Geometry: final body of the model. Coordinates: model frame, mm. A direction names the side the tool comes from. Coordinates: 2 decimals unless noted, no trailing zeros. Order: outer loops, then holes, each group sorted by start corner. A loop starts at its lowest first (then second) coordinate and runs counter-clockwise, first axis right, second up. Notation, with made-up numbers: (35.5, 24) - (40.5, 24) arc R20 ccw to (40.5, 60) - close; hole circle Ø6 at (-36.75, -9.5). An arc over 180 degrees is marked (long way). Use a Markdown table: item, result. Add a question column.
```python
from build123d import *

# Parameters (mm, degrees)
BOSS_EXTRUDE1_DEPTH = 3.175
VARFILLET1_START    = -1
VARFILLET1_DEPTH    = 5
VARFILLET2_DEPTH    = 3.175
SKETCH5_R           = 25.4
CUT_EXTRUDE1_DEPTH  = 3.175
SKETCH5_11_R        = 26.9875
SKETCH5_11_R_2      = 25.4
CUT_EXTRUDE2_DEPTH  = 0.9906
SKETCH24_R          = 11.1125
SKETCH24_R_2        = 7.9375
CUT_EXTRUDE5_DEPTH  = 0.9906
SKETCH24_2_R        = 7.9375
CUT_EXTRUDE6_DEPTH  = 3.175
SKETCH32_R          = 3.175
SKETCH32_R_2        = 3.2639
CUT_EXTRUDE10_DEPTH = 3.175
CIRPATTERN1_COUNT   = 3


with BuildPart() as part:
    # Basic Outline → Boss-Extrude1 (new body)
    with BuildSketch(Plane.XY):
        with BuildLine():
            Line((-38.1, 98.7206881), (-38.1, 21.997045256))
            Line((-38.1, 21.997045256), (-104.544623774, -16.364776166))
            ThreePointArc((-104.544623774, -16.364776166), (-76.653488005, -44.255911934), (-66.444623774, -82.355911934))
            Line((-66.444623774, -82.355911934), (0, -43.994090512))
            Line((0, -43.994090512), (66.444623774, -82.355911934))
            ThreePointArc((66.444623774, -82.355911934), (76.653488005, -44.255911934), (104.544623774, -16.364776166))
            Line((104.544623774, -16.364776166), (38.1, 21.997045256))
            Line((38.1, 21.997045256), (38.1, 98.7206881))
            ThreePointArc((38.1, 98.7206881), (0, 88.511823868), (-38.1, 98.7206881))
        make_face()
    extrude(amount=BOSS_EXTRUDE1_DEPTH)

    # VarFillet1: read off the stored shape, not the designer's step
    # VarFillet1 outline → VarFillet1 (cut)
    with BuildSketch(Plane.XY.offset(VARFILLET1_START)):
        with BuildLine():
            Line((-38.1, 98.7206881), (-38.1, 93.43325065))
            add(Edge.make_bspline(
                [(-38.1, 93.43325065), (-38.1, 98.524577309), (-33.528, 96.284393579)],
                knots=[0, 0, 0, 1, 1, 1], degree=2, weights=[1, 0.529150262, 1]))
            ThreePointArc((-33.528, 96.284393579), (-35.83471053, 97.463675037), (-38.1, 98.7206881))
        make_face()
        with BuildLine():
            ThreePointArc((38.1, 98.7206881), (35.83471053, 97.463675037), (33.528, 96.284393579))
            add(Edge.make_bspline(
                [(33.528, 96.284393579), (38.1, 98.524577309), (38.1, 93.43325065)],
                knots=[0, 0, 0, 1, 1, 1], degree=2, weights=[1, 0.529150262, 1]))
            Line((38.1, 93.43325065), (38.1, 98.7206881))
        make_face()
        with BuildLine():
            add(Edge.make_bspline(
                [(-100.148730828, -19.106097052), (-104.374786847, -16.26672077), (-99.965568621, -13.721057441)],
                knots=[0, 0, 0, 1, 1, 1], degree=2, weights=[1, 0.529150262, 1]))
            Line((-99.965568621, -13.721057441), (-104.544623774, -16.364776166))
            ThreePointArc((-104.544623774, -16.364776166), (-102.323373793, -17.698067863), (-100.148730828, -19.106097052))
        make_face()
        with BuildLine():
            add(Edge.make_bspline(
                [(-61.865568621, -79.712193209), (-66.274786847, -82.257856539), (-66.620730828, -77.178296528)],
                knots=[0, 0, 0, 1, 1, 1], degree=2, weights=[1, 0.529150262, 1]))
            ThreePointArc((-66.620730828, -77.178296528), (-66.488663264, -79.765607174), (-66.444623774, -82.355911934))
            Line((-66.444623774, -82.355911934), (-61.865568621, -79.712193209))
        make_face()
        with BuildLine():
            Line((104.544623774, -16.364776166), (99.965568621, -13.721057441))
            add(Edge.make_bspline(
                [(99.965568621, -13.721057441), (104.374786847, -16.26672077), (100.148730828, -19.106097052)],
                knots=[0, 0, 0, 1, 1, 1], degree=2, weights=[1, 0.529150262, 1]))
            ThreePointArc((100.148730828, -19.106097052), (102.323373793, -17.698067863), (104.544623774, -16.364776166))
        make_face()
        with BuildLine():
            ThreePointArc((66.444623774, -82.355911934), (66.488663264, -79.765607174), (66.620730828, -77.178296528))
            add(Edge.make_bspline(
                [(66.620730828, -77.178296528), (66.274786847, -82.257856539), (61.865568621, -79.712193209)],
                knots=[0, 0, 0, 1, 1, 1], degree=2, weights=[1, 0.529150262, 1]))
            Line((61.865568621, -79.712193209), (66.444623774, -82.355911934))
        make_face()
    extrude(amount=VARFILLET1_DEPTH, mode=Mode.SUBTRACT)

    # VarFillet2: read off the stored shape, not the designer's step
    # VarFillet2 outline → VarFillet2 (add)
    with BuildSketch(Plane.XY):
        with BuildLine():
            add(Edge.make_bspline(
                [(6.35, -47.660264722), (0, -43.994090512), (-6.35, -47.660264722)],
                knots=[0, 0, 0, 1, 1, 1], degree=2, weights=[1, 0.866025404, 1]))
            Line((6.35, -47.660264722), (0, -43.994090512))
            Line((0, -43.994090512), (-6.35, -47.660264722))
        make_face()
        with BuildLine():
            add(Edge.make_bspline(
                [(-44.45, 18.330871047), (-38.1, 21.997045256), (-38.1, 29.329393675)],
                knots=[0, 0, 0, 1, 1, 1], degree=2, weights=[1, 0.866025404, 1]))
            Line((-44.45, 18.330871047), (-38.1, 21.997045256))
            Line((-38.1, 21.997045256), (-38.1, 29.329393675))
        make_face()
        with BuildLine():
            add(Edge.make_bspline(
                [(38.1, 29.329393675), (38.1, 21.997045256), (44.45, 18.330871047)],
                knots=[0, 0, 0, 1, 1, 1], degree=2, weights=[1, 0.866025404, 1]))
            Line((38.1, 29.329393675), (38.1, 21.997045256))
            Line((38.1, 21.997045256), (44.45, 18.330871047))
        make_face()
    extrude(amount=VARFILLET2_DEPTH)

    # Sketch5 → Cut-Extrude1 (cut)
    with BuildSketch(Plane.XY.offset(3.175)):
        Circle(SKETCH5_R)
    extrude(amount=-CUT_EXTRUDE1_DEPTH, mode=Mode.SUBTRACT)

    # Sketch5_11 → Cut-Extrude2 (cut)
    with BuildSketch(Plane.XY.offset(3.175)):
        Circle(SKETCH5_11_R)
        Circle(SKETCH5_11_R_2, mode=Mode.SUBTRACT)
    extrude(amount=-CUT_EXTRUDE2_DEPTH, mode=Mode.SUBTRACT)

    # Sketch24 → Cut-Extrude5 (cut)
    # profile 1 of 3: a face of its own
    with BuildSketch(Plane.XY.offset(3.175)):
        with Locations((0, 50.8)):
            Circle(SKETCH24_R)
        with Locations((0, 50.8)):
            Circle(SKETCH24_R_2, mode=Mode.SUBTRACT)
    # profile 2 of 3: a face of its own
    with BuildSketch(Plane.XY.offset(3.175)):
        with Locations((-43.994090512, -25.4)):
            Circle(SKETCH24_R)
        with Locations((-43.994090512, -25.4)):
            Circle(SKETCH24_R_2, mode=Mode.SUBTRACT)
    # profile 3 of 3: a face of its own
    with BuildSketch(Plane.XY.offset(3.175)):
        with Locations((43.994090512, -25.4)):
            Circle(SKETCH24_R)
        with Locations((43.994090512, -25.4)):
            Circle(SKETCH24_R_2, mode=Mode.SUBTRACT)
    extrude(amount=-CUT_EXTRUDE5_DEPTH, mode=Mode.SUBTRACT)

    # Sketch24_2 → Cut-Extrude6 (cut)
    with BuildSketch(Plane.XY.offset(3.175)):
        with Locations((0, 50.8)):
            Circle(SKETCH24_2_R)
        with Locations((-43.994090512, -25.4)):
            Circle(SKETCH24_2_R)
        with Locations((43.994090512, -25.4)):
            Circle(SKETCH24_2_R)
    extrude(amount=-CUT_EXTRUDE6_DEPTH, mode=Mode.SUBTRACT)

    # Sketch32 → Cut-Extrude10 (cut)
    with BuildSketch(Plane.XY.offset(3.175)):
        with Locations((-31.877, 87.21025065)):
            Circle(SKETCH32_R)
        with Locations((-25.4, 80.73325065)):
            Circle(SKETCH32_R_2)
        with Locations((31.877, 87.21025065)):
            Circle(SKETCH32_R)
        with Locations((25.4, 80.73325065)):
            Circle(SKETCH32_R_2)
    cut_extrude10 = extrude(amount=-CUT_EXTRUDE10_DEPTH, mode=Mode.SUBTRACT)

    # CirPattern1: Cut-Extrude10 ×3 about axis
    cirpattern1_axis = Axis((0, 0, 0), (0, 0, 1))
    for i in range(1, CIRPATTERN1_COUNT):
        add(cut_extrude10.rotate(cirpattern1_axis, i * 360 / CIRPATTERN1_COUNT), mode=Mode.SUBTRACT)


solid = part.part
```
1) Set-up query: faces 1 (the face through (29.357, 85.278, 1.61)), 2 (the face through (-19.89, 18.24, 2.69)). Return all of +Z, -Z, +X, -X, +Y, -Y with unobstructed straight access to the full face (end or side cutting, diameter ignored); none if empty.
2) Section B-B (x = -14.5). Return loops of the section in (y, z) (1 decimal).
3) Ray query, line 1 along X through (y, z) = (81, 1.85); line 2 along Y through (x, z) = (0, 0.65); line 3 along Y through (x, z) = (-2, 1.9). Return the intervals inside material, ascending.
4) Draft query along Y for faces 3 (the face through (-76.898, -43.836, 1.565)), 4 (the face through (24, -10, 0)), 5 (the face through (27.15, 83.49, 1.61)), 6 (the face through (32.892, -24.911, 2.687)). Return one class per face: pulls with the +Y half, pulls with the -Y half, needs draft (parallel to the pull), parting line crosses it, or undercut.
5) Section A-A (y = 50.8). Return loops of the section in (x, z) (1 decimal).
6) Pin query (flat end, axial travel): pin 1 (1.5 mm diameter, centred on y = 57.5, z = 0.5, fed in from +X); pin 2 (4 mm diameter, centred on x = 82.62, y = -18.37, fed in from +Z). Return the tip coordinate at first contact, or that it passes through.
7) Section C-C (z = 0.6). Give the number of separate pieces and of enclosed holes in the cut face, then the cut area to 3 significant figures.
Values follow:
| question | item | result |
|---|---|---|
| 1 | face 1 | +Z, -Z |
| 1 | face 2 | +Z |
| 2 | outline | (-52.4, 0) - (-20.9, 0) - (-20.9, 2.2) - (-22.8, 2.2) - (-22.8, 3.2) - (-52.4, 3.2) - close; (20.9, 0) - (89.9, 0) - (89.9, 3.2) - (22.8, 3.2) - (22.8, 2.2) - (20.9, 2.2) - close |
| 3 | line 1 | x = -38.1 to -28.65, -22.15 to 22.15, 28.65 to 38.1 |
| 3 | line 2 | y = -45.96 to -25.4, 25.4 to 42.86, 58.74 to 88.51 |
| 3 | line 3 | y = -46.12 to -25.32, 25.32 to 43.12, 58.48 to 88.54 |
| 4 | face 3 | pulls with the -Y half |
| 4 | face 4 | needs draft |
| 4 | face 5 | undercut |
| 4 | face 6 | undercut |
| 5 | outline | (-38.1, 0) - (-7.9, 0) - (-7.9, 2.2) - (-11.1, 2.2) - (-11.1, 3.2) - (-38.1, 3.2) - close; (7.9, 0) - (38.1, 0) - (38.1, 3.2) - (11.1, 3.2) - (11.1, 2.2) - (7.9, 2.2) - close |
| 6 | pin 1 | stops at x = 38.1 |
| 6 | pin 2 | passes through |
| 7 | separate pieces | 1 |
| 7 | enclosed holes | 16 |
| 7 | area | 15,500 mm² |
